Geometry check sheet. Reference: the model listing, model coordinates, mm. Face numbers are marked on the shaded views. A direction names the side the tool comes from. Round coordinates to 2 decimals unless told otherwise and drop trailing zeros. Write each loop counter-clockwise with the first axis right and the second up, starting at its lowest first coordinate (ties: lowest second). Pieces come first, ordered by that corner, then holes.
Item 1: Access from +Z, -Z, +X, -X, +Y, -Y to the whole of each face (thin tool, end or side, straight path). Record for the marked faces 5, 6 and 7.
Item 2: Cross-section at B-B (x = 28). Enter the section's corners in (y, z).
Item 3: Depth check by flat-ended pin: P1, Ø2, axis at x = -1, z = 3, coming from the -Y side; P2, Ø1.5, axis at x = 18, z = 2.5, coming from the +Y side; P3, Ø1.5, axis at y = 6.5, z = 2.5, coming from the -X side. Enter the tip coordinate at first touch or a pass-through.
Item 4: Scan lines: probe 1 along Y at (x, z) = (30.75, 1.55); probe 2 along X at (y, z) = (-10.25, 3.05); probe 3 along Y at (x, z) = (30, 0.85). Record each from-to range of solid material in increasing order.
Item 5: Cross-section at C-C (y = 9.25). Enter the section's corners in (x, z), then the cut area to 3 significant figures.
Item 6: Cross-section at A-A (z = 3.45). State how many separate pieces and enclosed holes the cut face has, then the cut area to 3 significant figures.
Item 7: Draft check along X on the marked faces 1, 2, 3 and 4. Enter one of: pulls with the +X half, pulls with the -X half, needs draft (parallel to the pull), parting line crosses it, or undercut.
from build123d import *

# Parameters (mm, degrees)
SKETCH1_R           = 1.75
BOSS_EXTRUDE1_DEPTH = 4


with BuildPart() as part:
    # Sketch1 → Boss-Extrude1 (new body)
    with BuildSketch(Plane.XY):
        with BuildLine():
            ThreePointArc((14.048088143, -4.085109489), (14.06038767, -4.04257326), (14.072558403, -4))
            Line((14.072558403, -4), (30.75, -4))
            ThreePointArc((30.75, -4), (34.75, 0), (30.75, 4))
            Line((30.75, 4), (14.072558403, 4))
            ThreePointArc((14.072558403, 4), (14.06038767, 4.04257326), (14.048088143, 4.085109489))
            ThreePointArc((14.048088143, 4.085109489), (12.712915648, 4.255390909), (11.377106712, 4.090176385))
            ThreePointArc((11.377106712, 4.090176385), (0, 12.09), (-11.377106712, 4.090176385))
            ThreePointArc((-11.377106712, 4.090176385), (-12.712915648, 4.255390909), (-14.048088143, 4.085109489))
            ThreePointArc((-14.048088143, 4.085109489), (-14.131494839, 3.78652263), (-14.208555951, 3.486235477))
            ThreePointArc((-14.208555951, 3.486235477), (-13.137403362, 2.671181194), (-11.897951627, 2.1463567))
            ThreePointArc((-11.897951627, 2.1463567), (-11.986568374, 1.578061664), (-12.048056748, 1.00619511))
            ThreePointArc((-12.048056748, 1.00619511), (-13.381109763, 0.820047291), (-14.626715284, 0.31))
            ThreePointArc((-14.626715284, 0.31), (-14.63, 0), (-14.626715284, -0.31))
            ThreePointArc((-14.626715284, -0.31), (-13.381109763, -0.820047291), (-12.048056748, -1.00619511))
            ThreePointArc((-12.048056748, -1.00619511), (-11.986568374, -1.578061664), (-11.897951627, -2.1463567))
            ThreePointArc((-11.897951627, -2.1463567), (-13.137403362, -2.671181194), (-14.208555951, -3.486235477))
            ThreePointArc((-14.208555951, -3.486235477), (-14.131494839, -3.78652263), (-14.048088143, -4.085109489))
            ThreePointArc((-14.048088143, -4.085109489), (-12.712915648, -4.255390909), (-11.377106712, -4.090176385))
            ThreePointArc((-11.377106712, -4.090176385), (-11.169703548, -4.626642697), (-10.937020765, -5.152637848))
            ThreePointArc((-10.937020765, -5.152637848), (-11.998404632, -5.980373095), (-12.82210701, -7.044889767))
            ThreePointArc((-12.82210701, -7.044889767), (-12.669951657, -7.315), (-12.51210701, -7.581825517))
            ThreePointArc((-12.51210701, -7.581825517), (-11.17835734, -7.400736668), (-9.930825655, -6.8954189))
            ThreePointArc((-9.930825655, -6.8954189), (-9.591641884, -7.359925677), (-9.230750012, -7.807775241))
            ThreePointArc((-9.230750012, -7.807775241), (-10.041734454, -8.882012453), (-10.561852666, -10.123446462))
            ThreePointArc((-10.561852666, -10.123446462), (-10.344972209, -10.344972209), (-10.123446462, -10.561852666))
            ThreePointArc((-10.123446462, -10.561852666), (-8.882012453, -10.041734454), (-7.807775241, -9.230750012))
            ThreePointArc((-7.807775241, -9.230750012), (-7.359925677, -9.591641884), (-6.8954189, -9.930825655))
            ThreePointArc((-6.8954189, -9.930825655), (-7.400736668, -11.17835734), (-7.581825517, -12.51210701))
            ThreePointArc((-7.581825517, -12.51210701), (-7.315, -12.669951657), (-7.044889767, -12.82210701))
            ThreePointArc((-7.044889767, -12.82210701), (-5.980373095, -11.998404632), (-5.152637848, -10.937020765))
            ThreePointArc((-5.152637848, -10.937020765), (-4.626642697, -11.169703548), (-4.090176385, -11.377106712))
            ThreePointArc((-4.090176385, -11.377106712), (-4.255390909, -12.712915648), (-4.085109489, -14.048088143))
            ThreePointArc((-4.085109489, -14.048088143), (-3.78652263, -14.131494839), (-3.486235477, -14.208555951))
            ThreePointArc((-3.486235477, -14.208555951), (-2.671181194, -13.137403362), (-2.1463567, -11.897951627))
            ThreePointArc((-2.1463567, -11.897951627), (-1.578061664, -11.986568374), (-1.00619511, -12.048056748))
            ThreePointArc((-1.00619511, -12.048056748), (-0.820047291, -13.381109763), (-0.31, -14.626715284))
            ThreePointArc((-0.31, -14.626715284), (0, -14.63), (0.31, -14.626715284))
            ThreePointArc((0.31, -14.626715284), (0.820047291, -13.381109763), (1.00619511, -12.048056748))
            ThreePointArc((1.00619511, -12.048056748), (1.578061664, -11.986568374), (2.1463567, -11.897951627))
            ThreePointArc((2.1463567, -11.897951627), (2.671181194, -13.137403362), (3.486235477, -14.208555951))
            ThreePointArc((3.486235477, -14.208555951), (3.78652263, -14.131494839), (4.085109489, -14.048088143))
            ThreePointArc((4.085109489, -14.048088143), (4.255390909, -12.712915648), (4.090176385, -11.377106712))
            ThreePointArc((4.090176385, -11.377106712), (4.626642697, -11.169703548), (5.152637848, -10.937020765))
            ThreePointArc((5.152637848, -10.937020765), (5.980373095, -11.998404632), (7.044889767, -12.82210701))
            ThreePointArc((7.044889767, -12.82210701), (7.315, -12.669951657), (7.581825517, -12.51210701))
            ThreePointArc((7.581825517, -12.51210701), (7.400736668, -11.17835734), (6.8954189, -9.930825655))
            ThreePointArc((6.8954189, -9.930825655), (7.359925677, -9.591641884), (7.807775241, -9.230750012))
            ThreePointArc((7.807775241, -9.230750012), (8.882012453, -10.041734454), (10.123446462, -10.561852666))
            ThreePointArc((10.123446462, -10.561852666), (10.344972209, -10.344972209), (10.561852666, -10.123446462))
            ThreePointArc((10.561852666, -10.123446462), (10.041734454, -8.882012453), (9.230750012, -7.807775241))
            ThreePointArc((9.230750012, -7.807775241), (9.591641884, -7.359925677), (9.930825655, -6.8954189))
            ThreePointArc((9.930825655, -6.8954189), (11.17835734, -7.400736668), (12.51210701, -7.581825517))
            ThreePointArc((12.51210701, -7.581825517), (12.669951657, -7.315), (12.82210701, -7.044889767))
            ThreePointArc((12.82210701, -7.044889767), (11.998404632, -5.980373095), (10.937020765, -5.152637848))
            ThreePointArc((10.937020765, -5.152637848), (11.169703548, -4.626642697), (11.377106712, -4.090176385))
            ThreePointArc((11.377106712, -4.090176385), (12.712915648, -4.255390909), (14.048088143, -4.085109489))
        make_face()
        Circle(SKETCH1_R, mode=Mode.SUBTRACT)
        with Locations((30.75, 0)):
            Circle(SKETCH1_R, mode=Mode.SUBTRACT)
    extrude(amount=BOSS_EXTRUDE1_DEPTH)


solid = part.part
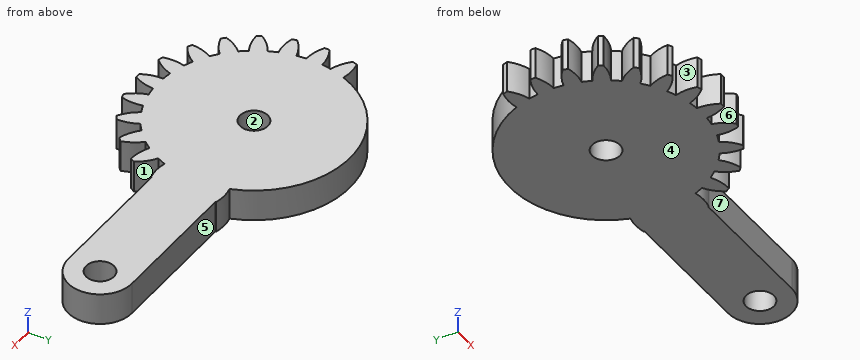
Resolved:
1. face 5: +Z, -Z, +X, +Y
1. face 6: +Z, -Z, -Y
1. face 7: +Z, -Z, +X, -Y
2. outline: (-4, 0) - (4, 0) - (4, 4) - (-4, 4) - close
3. P1: stops at y = -14.63
3. P2: stops at y = 4
3. P3: stops at x = -10.64
4. probe 1: y = -4 to -1.75, 1.75 to 4
4. probe 2: x = -10.44 to -9.28, -7.06 to 7.06, 9.28 to 10.44
4. probe 3: y = -4 to -1.58, 1.58 to 4
5. outline: (-7.78, 0) - (7.78, 0) - (7.78, 4) - (-7.78, 4) - close
5. area: 62.3 mm2
6. separate pieces: 1
6. enclosed holes: 2
6. area: 664 mm2
7. face 1: pulls with the +X half
7. face 2: undercut
7. face 3: undercut
7. face 4: needs draft
